Build history of the part. All positions in model axes, mm. Face numbers are marked on the shaded views. A direction names the side the tool comes from. Round coordinates to 2 decimals unless told otherwise and drop trailing zeros. Loops run counter-clockwise (first coordinate to the right, second up) from the corner with the lowest first, then second, coordinate; pieces in that order, holes last. Notation, with made-up numbers: (5, 79.5) - (55, 79.5) arc R21 ccw to (55, 102.5) - close; hole circle Ø7 at (85, -12). An arc over 180 degrees is marked (long way). Put each result on its own line as item: value. Start each with the question number.
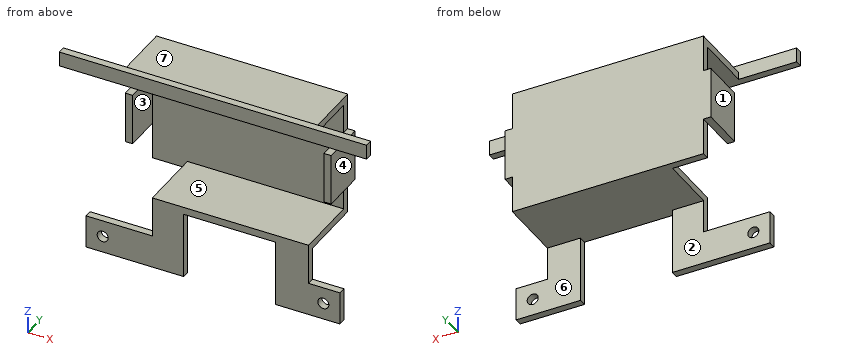
from build123d import *

# Parameters (mm, degrees)
SKETCH1_W            = 52
SKETCH1_H            = 34
BOSS_EXTRUDE1_DEPTH  = 19.65
SKETCH2_W            = 52
SKETCH2_H            = 30
CUT_EXTRUDE1_DEPTH   = 17.65
SKETCH3_W            = 9
SKETCH3_H            = 2
SKETCH3_W_2          = 18
BOSS_EXTRUDE2_DEPTH  = 18
SKETCH4_W            = 18
SKETCH4_H            = 2
BOSS_EXTRUDE3_DEPTH  = 8.5
SKETCH5_W            = 18
SKETCH5_H            = 2
BOSS_EXTRUDE4_DEPTH  = 8.5
SKETCH6_R            = 1.5
CUT_EXTRUDE2_DEPTH   = 82.705400678
SKETCH7_W            = 52
SKETCH7_H            = 2
BOSS_EXTRUDE5_DEPTH  = 2
SKETCH8_W            = 4
SKETCH8_H            = 2
BOSS_EXTRUDE6_DEPTH  = 15.78
SKETCH9_W            = 4
SKETCH9_H            = 2
BOSS_EXTRUDE7_DEPTH  = 15.78
SKETCH11_W           = 11
SKETCH11_H           = 17.65
CUT_EXTRUDE3_DEPTH   = 18
SKETCH12_W           = 9
SKETCH12_H           = 2
CUT_EXTRUDE4_DEPTH   = 8.5
SKETCH14_W           = 14
SKETCH14_H           = 2
BOSS_EXTRUDE8_DEPTH  = 2
SKETCH15_W           = 14
SKETCH15_H           = 2
BOSS_EXTRUDE9_DEPTH  = 2
SKETCH16_W           = 2
SKETCH16_H           = 14
BOSS_EXTRUDE10_DEPTH = 10


with BuildPart() as part:
    # Sketch1 → Boss-Extrude1 (new body)
    with BuildSketch(Plane(origin=(0, 0, 0), x_dir=(1, 0, 0), z_dir=(0, 1, 0))):
        with Locations((26, 17)):
            Rectangle(SKETCH1_W, SKETCH1_H)
    extrude(amount=BOSS_EXTRUDE1_DEPTH)

    # Sketch2 → Cut-Extrude1 (cut)
    with BuildSketch(Plane(origin=(0, 0, 0), x_dir=(-1, 0, 0), z_dir=(0, -1, 0))):
        with Locations((-26, 17)):
            Rectangle(SKETCH2_W, SKETCH2_H)
    extrude(amount=-CUT_EXTRUDE1_DEPTH, mode=Mode.SUBTRACT)

    # Sketch3 → Boss-Extrude2 (add)
    with BuildSketch(Plane(origin=(0, 0, -34), x_dir=(-1, 0, 0), z_dir=(0, 0, -1))):
        with Locations((-47.5, 1)):
            Rectangle(SKETCH3_W, SKETCH3_H)
        with Locations((-9, 1)):
            Rectangle(SKETCH3_W_2, SKETCH3_H)
    extrude(amount=BOSS_EXTRUDE2_DEPTH)

    # Sketch4 → Boss-Extrude3 (add)
    with BuildSketch(Plane(origin=(52, 0, 0), x_dir=(0, 0, -1), z_dir=(1, 0, 0))):
        with Locations((43, 1)):
            Rectangle(SKETCH4_W, SKETCH4_H)
    extrude(amount=BOSS_EXTRUDE3_DEPTH)

    # Sketch5 → Boss-Extrude4 (add)
    with BuildSketch(Plane.ZY):
        with Locations((-43, 1)):
            Rectangle(SKETCH5_W, SKETCH5_H)
    extrude(amount=BOSS_EXTRUDE4_DEPTH)

    # Sketch6 → Cut-Extrude2 (cut, through all)
    with BuildSketch(Plane(origin=(0, 2, 0), x_dir=(1, 0, 0), z_dir=(0, 1, 0))):
        with Locations(Location((56, 47.5, 0), (0, 0, 270))):
            Circle(SKETCH6_R)
        with Locations(Location((-4, 47.5, 0), (0, 0, 270))):
            Circle(SKETCH6_R)
    extrude(amount=-CUT_EXTRUDE2_DEPTH, mode=Mode.SUBTRACT)

    # Sketch7 → Boss-Extrude5 (add)
    with BuildSketch(Plane.XY):
        with Locations((26, 1)):
            Rectangle(SKETCH7_W, SKETCH7_H)
    extrude(amount=BOSS_EXTRUDE5_DEPTH)

    # Sketch8 → Boss-Extrude6 (add)
    with BuildSketch(Plane.ZY):
        with Locations((0, 1)):
            Rectangle(SKETCH8_W, SKETCH8_H)
    extrude(amount=BOSS_EXTRUDE6_DEPTH)

    # Sketch9 → Boss-Extrude7 (add)
    with BuildSketch(Plane(origin=(52, 0, 0), x_dir=(0, 0, -1), z_dir=(1, 0, 0))):
        with Locations((0, 1)):
            Rectangle(SKETCH9_W, SKETCH9_H)
    extrude(amount=BOSS_EXTRUDE7_DEPTH)

    # Sketch11 → Cut-Extrude3 (cut)
    with BuildSketch(Plane.ZY.offset(8.5)):
        with Locations((-37.5, 8.825)):
            Rectangle(SKETCH11_W, SKETCH11_H)
    extrude(amount=-CUT_EXTRUDE3_DEPTH, mode=Mode.SUBTRACT)

    # Sketch12 → Cut-Extrude4 (cut)
    with BuildSketch(Plane(origin=(60.5, 0, 0), x_dir=(0, 0, -1), z_dir=(1, 0, 0))):
        with Locations((38.5, 1)):
            Rectangle(SKETCH12_W, SKETCH12_H)
    extrude(amount=-CUT_EXTRUDE4_DEPTH, mode=Mode.SUBTRACT)

    # Sketch14 → Boss-Extrude8 (add)
    with BuildSketch(Plane.ZY):
        with Locations((-17, 18.65)):
            Rectangle(SKETCH14_W, SKETCH14_H)
    extrude(amount=BOSS_EXTRUDE8_DEPTH)

    # Sketch15 → Boss-Extrude9 (add)
    with BuildSketch(Plane(origin=(52, 0, 0), x_dir=(0, 0, -1), z_dir=(1, 0, 0))):
        with Locations((17, 18.65)):
            Rectangle(SKETCH15_W, SKETCH15_H)
    extrude(amount=BOSS_EXTRUDE9_DEPTH)

    # Sketch16 → Boss-Extrude10 (add)
    with BuildSketch(Plane(origin=(0, 17.65, 0), x_dir=(-1, 0, 0), z_dir=(0, -1, 0))):
        with Locations((1, 17)):
            Rectangle(SKETCH16_W, SKETCH16_H)
        with Locations((-53, 17)):
            Rectangle(SKETCH16_W, SKETCH16_H)
    extrude(amount=BOSS_EXTRUDE10_DEPTH)


solid = part.part
Item 1: Two-plate mould, pull along X, no slides. Class the marked faces 1, 2, 3 and 4: pulls with the +X half, pulls with the -X half, needs draft (parallel to the pull), parting line crosses it, or undercut.
Item 2: Slice it at B-B (z = -47.5). Give the cut face in (x, y), plus the area to 3 significant figures.
Item 3: Slice it at C-C (y = 11.25). Give the cut face in (x, z), plus the area to 3 significant figures.
Item 4: Drop flat-ended pins along their axis: pin 1 Ø9 at (x, z) = (-1, -45) entering from +Y; pin 2 Ø1.8 at (x, z) = (-4, -47.5) entering from +Y; pin 3 Ø10 at (x, y) = (47, 13) entering from +Z; pin 4 Ø1.6 at (x, y) = (52.5, 13.5) entering from -Z. Give the stop position or say it passes through.
Item 5: Slice it at D-D (z = -22.5). Give the cut face in (x, y).
Item 6: Drill centre lines: probe 1 along X at (y, z) = (1, -47.5); probe 2 along Z at (x, y) = (37.5, 16); probe 3 along X at (y, z) = (11.75, -22). Where is each one in solid material? Low to high. Write a range as [from, to].
Item 7: Slice it at A-A (x = 56). Give the cut face in (y, z).
Item 8: Which spindle directions (+Z, -Z, +X, -X, +Y, -Y) get a long thin tool onto all of the face, cutting with end or side? Do the marked faces 5, 6 and 7. Say none if no direction does.
Computed values:
1. face 1: pulls with the -X half
1. face 2: needs draft
1. face 3: undercut
1. face 4: pulls with the +X half
2. outline: (-8.5, 0) - (-5.5, 0) - (-5.5, 2) - (-8.5, 2) - close; (-2.5, 0) - (18, 0) - (18, 2) - (-2.5, 2) - close; (43, 0) - (54.5, 0) - (54.5, 2) - (43, 2) - close; (57.5, 0) - (60.5, 0) - (60.5, 2) - (57.5, 2) - close
2. area: 76.0 mm^2
3. outline: (-2, -24) - (0, -24) - (0, -10) - (-2, -10) - close; (0, -2) - (52, -2) - (52, 0) - (0, 0) - close; (9.5, -34) - (52, -34) - (52, -32) - (9.5, -32) - close; (52, -24) - (54, -24) - (54, -10) - (52, -10) - close
3. area: 245 mm^2
4. pin 1: stops at y = 2
4. pin 2: passes through
4. pin 3: stops at z = 0
4. pin 4: stops at z = -34
5. outline: (-2, 7.65) - (0, 7.65) - (0, 17.65) - (52, 17.65) - (52, 7.65) - (54, 7.65) - (54, 19.65) - (-2, 19.65) - close
6. probe 1: x = [-8.5, -5.5], [-2.5, 18], [43, 54.5], [57.5, 60.5]
6. probe 2: z = [-34, -32], [-2, 0]
6. probe 3: x = [-2, 0], [52, 54]
7. outline: (0, -52) - (2, -52) - (2, -49) - (0, -49) - close; (0, -46) - (2, -46) - (2, -43) - (0, -43) - close; (0, -2) - (2, -2) - (2, 2) - (0, 2) - close
8. face 5: +X, -X, -Y
8. face 6: -Z, +X, -X, +Y
8. face 7: +Z, +X, -X, +Y
